from build123d import *

# Parameters (mm, degrees)
F1_DEPTH = 15.24
F2_R     = 5.08
F5_D     = 4.699


with BuildPart() as f1:
    # F0 (on Front) → F1 (new body)
    with BuildSketch(Plane.XZ):
        with BuildLine():
            Line((53.34, 25.4), (-53.34, 25.4))
            ThreePointArc((-53.34, 25.4), (-59.626179, 22.796179), (-62.23, 16.51))
            Line((-62.23, 16.51), (-62.23, 7.9248))
            ThreePointArc((-62.23, 7.9248), (-62.973949, 6.128749), (-64.77, 5.3848))
            Line((-64.77, 5.3848), (-74.6125, 5.3848))
            Line((-74.6125, 5.3848), (-74.6125, 0))
            Line((-74.6125, 0), (-66.04, 0))
            ThreePointArc((-66.04, 0), (-59.753821, 2.603821), (-57.15, 8.89))
            Line((-57.15, 8.89), (-57.15, 13.1318))
            ThreePointArc((-57.15, 13.1318), (-55.662102, 16.723902), (-52.07, 18.2118))
            Line((-52.07, 18.2118), (52.07, 18.2118))
            ThreePointArc((52.07, 18.2118), (55.662102, 16.723902), (57.15, 13.1318))
            Line((57.15, 13.1318), (57.15, 8.89))
            ThreePointArc((57.15, 8.89), (59.753821, 2.603821), (66.04, 0))
            Line((66.04, 0), (74.6125, 0))
            Line((74.6125, 0), (74.6125, 5.3848))
            Line((74.6125, 5.3848), (64.77, 5.3848))
            ThreePointArc((64.77, 5.3848), (62.973949, 6.128749), (62.23, 7.9248))
            Line((62.23, 7.9248), (62.23, 16.51))
            ThreePointArc((62.23, 16.51), (59.626179, 22.796179), (53.34, 25.4))
        make_face()
    extrude(amount=F1_DEPTH)

    # F2
    f2_edges = [f1.edges().sort_by_distance(p)[0] for p in [
        (-74.6125, -15.24, 2.6924),
        (74.6125, -15.24, 2.6924),
    ]]
    fillet(f2_edges, radius=F2_R)

    # F5 (through all)
    with Locations(Plane.XY.offset(5.3848)):
        with Locations((-69.69125, -7.62), (69.69125, -7.62)):
            Hole(F5_D / 2)


solid = f1.part
Build history of the part. All positions in model axes, mm. A direction names the side the tool comes from. Coordinates: 2 decimals unless noted, no trailing zeros. Order: outer loops, then holes, each group sorted by start corner. A loop starts at its lowest first (then second) coordinate and runs counter-clockwise, first axis right, second up. Notation, with made-up numbers: (35.5, 48) - (80.5, 48) arc R17 ccw to (80.5, 56) - close; hole circle Ø10 at (44, 85.25). An arc over 180 degrees is marked (long way). Write each question's results on one line, items separated by ' | '. Start each with the question number.
Item 1: Mould opens along Y. For faces 1 (the face through (-59.56, -7.51, 22.86)), 2 (the face through (67.45, -6.91, 2.65)), 3 (the face through (0, -15.24, 20)) say: released by +Y, released by -Y, zero draft, split by the parting line, or undercut.
Item 2: Band-saw the part on B-B on y = -7.62. Write the cut outline in (x, z).
Item 3: Flat gauge pins, fed straight in: pin 1 (8 mm diameter, centred on x = 68, y = -4.5, fed in from +Z); pin 2 (2 mm diameter, centred on y = -6, z = 7.5, fed in from +X); pin 3 (5 mm diameter, centred on y = -8.5, z = 10, fed in from +X); pin 4 (4 mm diameter, centred on x = 69.69, y = -7.62, fed in from -Z). Where does each tip first touch, or does it go through?
Item 4: Band-saw the part on C-C on x = 30.5. Write the cut outline in (y, z), and give its area (3 significant figures).
Item 5: Band-saw the part on A-A on z = 3. Write the cut outline in (x, y).
Item 6: Wall check: probe 1 along X at (y, z) = (-2, 8.25); probe 2 along Z at (x, y) = (-26, -5.25); probe 3 along X at (y, z) = (-7, 15). Give the ranges that are in metal, low to high. Write a range as [from, to].
Item 7: Band-saw the part on D-D on z = 20. Write the cut outline in (x, y).
Item 8: Tool access for faces 4 (the face through (67.6, -5.8, 5.385)), 5 (the face through (55.622, -7.513, 16.763)), 6 (the face through (-67, -6, 5.385)): list every direction of +Z, -Z, +X, -X, +Y, -Y with a clear straight run to the whole face (end or side of a thin tool).
Numbers:
1) face 1: zero draft | face 2: undercut | face 3: released by -Y
2) outline: (-74.61, 0) - (-72.04, 0) - (-72.04, 5.38) - (-74.61, 5.38) - close; (-67.34, 0) - (-66.04, 0) arc R8.89 ccw to (-57.15, 8.89) - (-57.15, 13.13) arc R5.08 cw to (-52.07, 18.21) - (52.07, 18.21) arc R5.08 cw to (57.15, 13.13) - (57.15, 8.89) arc R8.89 ccw to (66.04, 0) - (67.34, 0) - (67.34, 5.38) - (64.77, 5.38) arc R2.54 cw to (62.23, 7.92) - (62.23, 16.51) arc R8.89 ccw to (53.34, 25.4) - (-53.34, 25.4) arc R8.89 ccw to (-62.23, 16.51) - (-62.23, 7.92) arc R2.54 cw to (-64.77, 5.38) - (-67.34, 5.38) - close; (72.04, 0) - (74.61, 0) - (74.61, 5.38) - (72.04, 5.38) - close
3) pin 1: z = 5.5 | pin 2: x = 62.67 | pin 3: x = 62.27 | pin 4: through
4) outline: (-15.24, 18.21) - (0, 18.21) - (0, 25.4) - (-15.24, 25.4) - close | area: 110 mm^2
5) outline: (-74.61, -10.16) arc R5.08 ccw to (-69.53, -15.24) - (-59.38, -15.24) - (-59.38, 0) - (-74.61, 0) - close; (59.38, -15.24) - (69.53, -15.24) arc R5.08 ccw to (74.61, -10.16) - (74.61, 0) - (59.38, 0) - close; hole circle Ø4.7 at (-69.69, -7.62); hole circle Ø4.7 at (69.69, -7.62)
6) probe 1: [-62.23, -57.17], [57.17, 62.23] | probe 2: [18.21, 25.4] | probe 3: [-62.23, -56.79], [56.79, 62.23]
7) outline: (-61.52, -15.24) - (61.52, -15.24) - (61.52, 0) - (-61.52, 0) - close
8) face 4: +Z, +X, +Y, -Y | face 5: -Z, +Y, -Y | face 6: +Z, -X, +Y, -Y
